Autodesk Inventor part; units mm, degrees
ref_plane "Work Plane1" through (-166.5525, 2.666, -98.7961) normal (0, 0, -1) x (-1, 0, 0)
ref_plane "Work Plane2" through (-38.4044, -9.834, -118.7961) normal (0, -1, 0) x (1, 0, 0)
ref_plane "Work Plane3" through (-25.7044, 2.666, -220.3961) normal (0, -1, 0) x (1, 0, 0)
ref_plane "Work Plane1" through (-166.5525, 2.666, -98.7961) normal (0, 0, -1) x (-1, 0, 0)
sketch "Sketch1" plane through (-166.5525, 2.666, -98.7961) normal (0, 0, -1) x (-1, 0, 0)
  line L0 (-233.1482, 205) -> (-133.1482, 205)
  line L1 (-133.1482, 205) -> (-133.1482, -25)
  line L2 (-133.1482, -25) -> (-233.1482, -25)
  line L3 (-233.1482, -25) -> (-233.1482, 205)
  circle A0 centre (0, 0) radius 140
  circle A1 centre (-210, 25) radius 2.4585
  circle A2 centre (-185, 25) radius 2.4585
  circle A3 centre (-160, 25) radius 2.4585
  circle A4 centre (-185, 0) radius 2.4585
  circle A5 centre (-210, 0) radius 2.4585
  circle A6 centre (-160, 0) radius 2.4585
  circle A7 centre (0.3518, 0) radius 128.5
  line L4 (-128.1482, 39.0483) -> (-128.1482, -22.9652) construction
  dimension "d10" = 5
  dimension "d56" = 230
  dimension "d57" = 100
  dimension "d63" = 25
extrude "Extrusion1" add sketch "Sketch1" along normal blind 10 contours L0 L1 A0 L2 L3 | L1 L2 A0 | A1 | A2 | A3 | A4 | A5 | A6 picked at (-134.3536, 16.0623)
hole "Hole1" at (43.4475, 27.666, -108.7961) at (18.4475, 27.666, -108.7961) at (-6.5525, 27.666, -108.7961) at (43.4475, 2.666, -108.7961) at (18.4475, 2.666, -108.7961) at (-6.5525, 2.666, -108.7961) direction (0, 0, 1) diameter 6.6 end through all counterbore diameter 11 counterbore depth 6.8
ref_plane "Work Plane2" through (-38.4044, -9.834, -118.7961) normal (0, -1, 0) x (1, 0, 0)
sketch "Sketch3" plane through (-38.4044, -9.834, -118.7961) normal (0, -1, 0) x (1, 0, 0)
  line L0 (5, 10) -> (55, 10)
  line L1 (55, 10) -> (55, -75)
  line L2 (50, -80) -> (32.7284, -80)
  line L3 (5, -35.6333) -> (5, 10)
  line L4 (105, 10) -> (5, 10)
  line L5 (5, 20) -> (5, 10)
  circle A0 centre (22.225, -22.225) radius 12.7
  circle A1 centre (22.225, -22.225) radius 10
  line L6 (5.6699, -38.1333) -> (28.3983, -77.5)
  line L7 (5, -36.973) -> (50.4568, -36.973) construction
  arc A2 (28.3983, -77.5) -> (32.7284, -80) centre (32.7284, -75) ccw
  arc A3 (50, -80) -> (55, -75) centre (50, -75) ccw
  arc A4 (5, -35.6333) -> (5.6699, -38.1333) centre (10, -35.6333) ccw
  point P0 (38.4044, 118.7961)
  dimension "d11" = 20
  dimension "d13" = 60
  dimension "d14" = 5
  dimension "d58" = 90
  dimension "d60" = 50
extrude "Extrusion2" add sketch "Sketch3" along normal mid plane 10 contours L0 L1 A3 L2 A2 L6 A4 L3 | A0
ref_plane "Work Plane3" through (-25.7044, 2.666, -220.3961) normal (0, -1, 0) x (1, 0, 0)
mirror "Mirror1" about plane through (-25.7044, 2.666, -220.3961) normal (0, -1, 0) of "Extrusion2"
sketch "Sketch4" plane through (-166.5525, 2.666, -108.7961) normal (0, 0, -1) x (-1, 0, 0)
  line L0 (-133.1482, 205) -> (-133.1482, -25)
  line L1 (-133.1482, 32.5) -> (-183.1482, 32.5)
  line L2 (-183.1482, 32.5) -> (-183.1482, 42.5)
  line L3 (-183.1482, 42.5) -> (-133.1482, 42.5)
  line L4 (-133.1482, 42.5) -> (-133.1482, 32.5)
  line L5 (-183.1482, 17.5) -> (-183.1482, 7.5)
  circle A0 centre (-185, 25) radius 3.3
  line L6 (-160.8766, 17.5) -> (-178.1482, 17.5)
  point P0 (-166.5525, -2.666)
  dimension "d17" = 4.2
  dimension "d18" = 4.2
  dimension "d19" = 10
extrude "Extrusion3" add sketch "Sketch4" along normal blind 50 contours L0 L1 L2 L3
fillet "Fillet1" radius 5 2 edges at (-33.4044, 40.166, -158.7961) (16.5956, 40.166, -158.7961)
sketch "Sketch5" plane through (-33.4044, 45.166, -108.7961) normal (0, 1, 0) x (1, 0, 0)
  circle A0 centre (17.225, 32.225) radius 10
  point P0 (33.4044, -108.7961)
extrude "Extrusion4" cut sketch "Sketch5" against normal blind 15.75
ref_plane "Work Plane6" through (-16.1794, 92.1501, -148.7711) normal (0, -1, 0) x (0, 0, 1)
sketch "Sketch7" plane through (-16.1794, 92.1501, -148.7711) normal (0, -1, 0) x (0, 0, 1)
  line L0 (39.975, 17.225) -> (39.975, -82.775)
  line L1 (39.975, 17.225) -> (-5.025, 17.225)
  line L2 (-10.025, 12.225) -> (-10.025, -12.775)
  line L3 (-5.025, -17.775) -> (39.975, -17.775)
  line L4 (39.975, -17.775) -> (39.975, 17.225)
  arc A0 (-5.025, 17.225) -> (-10.025, 12.225) centre (-5.025, 12.225) ccw
  arc A1 (-10.025, -12.775) -> (-5.025, -17.775) centre (-5.025, -12.775) ccw
  point P0 (148.7711, -16.1794)
  point P1 (-10.025, -17.775)
  point P2 (-10.025, 17.225)
  point P3 (7.75, 0)
  dimension "d25" = 50
  dimension "d26" = 35
  dimension "d27" = 5
extrude "Extrusion5" [suppressed]
sketch "Sketch8" plane through (-16.1794, 85.1501, -148.7711) normal (0, -1, 0) x (1, 0, 0)
  point P0 (16.1794, 148.7711)
  point P1 (0, 7.75)
hole "Hole2" [suppressed]
ref_plane "Work Plane8" through (-11.7294, 189.1501, -141.0211) normal (1, 0, 0) x (0, -1, 0)
sketch "Sketch12" plane through (-11.7294, 189.1501, -141.0211) normal (1, 0, 0) x (0, -1, 0)
  circle A0 centre (-2, 0) radius 2
  line L0 (0, 4.5164) -> (0, 7)
  line L1 (-9.233, 4.5164) -> (0, 4.5164)
  spline S0 degree 2 poles (-10, 3.4325) (-9.6688, 3.9374) (-9.233, 4.5164) knots 0 0 0 0.1328 0.1328 0.1328 weights 1 1.004688 1
  line L2 (-10, -3.4325) -> (-10, 3.4325)
  spline S1 degree 2 poles (-9.233, -4.5164) (-9.6688, -3.9374) (-10, -3.4325) knots 0 0 0 0.1328 0.1328 0.1328 weights 1 1.004688 1
  line L3 (0, -4.5164) -> (-9.233, -4.5164)
  line L4 (0, -7) -> (0, -4.5164)
  line L5 (0, -7) -> (4.2876, -7)
  spline S2 degree 2 poles (4, -6.6678) (4.1403, -6.8309) (4.2876, -7) knots 0 0 0 0.044596 0.044596 0.044596 weights 1 1.000378 1.000314
  line L6 (4, 6.6678) -> (4, -6.6678)
  spline S3 degree 2 poles (4.2876, 7) (4.1403, 6.8309) (4, 6.6678) knots 0.03161 0.03161 0.03161 0.076206 0.076206 0.076206 weights 1.000314 1.000378 1
  line L7 (-18.5159, -32.225) -> (211.4841, -32.225)
  line L8 (1.2341, 7.775) -> (-8.2659, 7.775)
  line L9 (-10.2659, 5.775) -> (-10.2659, -32.225)
  line L10 (-10.2659, -32.225) -> (3.2341, -32.225)
  line L11 (3.2341, -32.225) -> (3.2341, 5.775)
  arc A1 (-8.2659, 7.775) -> (-10.2659, 5.775) centre (-8.2659, 5.775) ccw
  arc A2 (3.2341, 5.775) -> (1.2341, 7.775) centre (1.2341, 5.775) ccw
  line L12 (-18.5159, -42.225) -> (-18.5159, -32.225)
  point P0 (189.1501, -141.0211)
  point P1 (3.2341, 7.775)
  point P2 (-3.5159, 7.775)
  dimension "d48" = 13.5
  dimension "d49" = 2
  dimension "d62" = 40
  dimension "d79" = 15
extrude "Extrusion7" add sketch "Sketch12" along normal blind 10
ref_plane "Work Plane10" through (-16.1794, 180.6501, -141.0211) normal (-1, 0, 0) x (0, 1, 0)
ref_plane "Work Plane9" through (-20.6294, 180.6501, -141.0211) normal (-1, 0, 0) x (0, 1, 0)
mirror "Mirror2" about plane through (-16.1794, 180.6501, -141.0211) normal (-1, 0, 0) of "Extrusion7"
sketch "Sketch13" plane through (-166.5525, 2.666, -108.7961) normal (0, 0, -1) x (-1, 0, 0)
  line L0 (-233.1482, 205) -> (-188.1482, 205)
  line L1 (-188.1482, 205) -> (-188.1482, 75)
  line L2 (-188.1482, 75) -> (-233.1482, 75)
  line L3 (-233.1482, 75) -> (-233.1482, 205)
  line L4 (-233.1482, -25) -> (-133.1482, -25)
  line L5 (-133.1482, 42.5) -> (-133.1482, 205)
  point P0 (-166.5525, -2.666)
  point P1 (-133.1482, 89.4841)
  dimension "d52" = 100
  dimension "d53" = 55
extrude "Extrusion8" [suppressed]
ref_plane "Work Plane11" through (-33.4044, 2.666, -108.7961) normal (0, -1, 0) x (1, 0, 0)
sketch "Sketch15" plane through (-166.5525, 2.666, -108.7961) normal (0, 0, -1) x (-1, 0, 0)
  line L0 (-133.1482, 205) -> (-133.1482, -25) construction
  line L1 (-133.1482, 95) -> (-183.1482, 95) construction
  line L2 (-133.1482, 95) -> (-83.1482, 95) construction
  line L3 (-133.1482, 205) -> (-233.1482, 205) construction
  line L4 (-183.1482, 91.5) -> (-133.1482, 91.5)
  line L5 (-133.1482, 91.5) -> (-133.1482, 98.5)
  line L6 (-133.1482, 98.5) -> (-183.1482, 98.5)
  line L7 (-183.1482, 98.5) -> (-183.1482, 91.5)
  line L8 (-183.1482, 91.5) -> (-133.1482, 98.5) construction
  line L9 (-133.1482, 91.5) -> (-183.1482, 98.5) construction
  point P0 (-166.5525, -2.666)
  point P1 (-158.1482, 95)
  dimension "d64" = 50
  dimension "d65" = 180
  dimension "d66" = 110
  dimension "d67" = 7
extrude "Extrusion9" add sketch "Sketch15" along normal blind 50
fillet "Fillet2" radius 5 2 edges at (-33.4044, 97.666, -158.7961) (16.5956, 97.666, -158.7961)
sketch "Sketch16" plane through (-33.4044, 101.166, -108.7961) normal (0, 1, 0) x (1, 0, 0)
  point P0 (33.4044, -108.7961)
  point P1 (17.225, 32.225)
hole "Hole3" at (-16.1794, 101.166, -141.0211) direction (0, -1, 0) diameter 12.2 depth 17.1 tip angle 118
equation "\"d18\" = d17"
properties part number "Verbinder_Tisch_Dewar"
Input: part model. Units: mm. Frame: model coordinates. A direction names the side the tool comes from. Coordinates: 2 decimals unless noted, no trailing zeros. Write each loop counter-clockwise with the first axis right and the second up, starting at its lowest first coordinate (ties: lowest second). Pieces come first, ordered by that corner, then holes. Notation, with made-up numbers: (44, 68) - (95, 68) arc R20 cw to (95, 101) - close; hole circle Ø2 at (-39, 88). An arc over 180 degrees is marked (long way). Put each result on its own line as item: value. Start each with the question number.
1) Mould query, pull axis Y, two halves, no side actions, for faces 6 (the face through (-3, -14.834, -153)), 7 (the face through (-8, 45.166, -133)), 8 (the face through (16.22, 0.23, -100.37)), 9 (the face through (-18.35, 40.24, -131.26)). Classes: pulls with the +Y half, pulls with the -Y half, needs draft (parallel to the pull), parting line crosses it, or undercut.
2) Cut plane C-C (x = 28). Return the cut outline in (y, z), plus the area to 3 significant figures.
3) Ray query, L1, parallel to Y at x = 5.5, z = -131; L2, parallel to Y at x = -7.5, z = -192; L3, parallel to X at y = 192, z = -147. Return the intervals inside material, ascending.
4) Contact query for flat-ended pins moving along their axis: pin 1 (10 mm diameter, centred on x = 50.5, y = 42, fed in from -Z); pin 2 (4 mm diameter, centred on y = 194, z = -120.5, fed in from -X); pin 3 (25 mm diameter, centred on x = -15.5, z = -123, fed in from +Y). Output: stop coordinate, or through.
5) Cut plane A-A (z = -125.5). Return the cut outline in (x, y), plus the area to 3 significant figures.
6) Reachability of faces 1 (the face through (-30.629, 193, -129)), 2 (the face through (46.79, -1.7, -105.35)), 3 (the face through (-18.35, 15.24, -131.26)), 4 (the face through (15.09, 97.62, -157.37)), 5 (the face through (-20.629, 193, -129)) from +Z, -Z, +X, -X, +Y, -Y: full face, straight path, thin tool, end or side. Return the list, or none.
7) Cut plane B-B (z = -189). Return the cut outline in (x, y), plus the area to 3 significant figures.
8) Cut plane D-D (z = -169). Return the cut outline in (x, y), plus the area to 3 significant figures.
Resolved:
1. face 6: pulls with the -Y half
1. face 7: undercut
1. face 8: undercut
1. face 9: needs draft
2. outline: (-22.33, -108.8) - (207.67, -108.8) - (207.67, -98.8) - (-22.33, -98.8) - close
2. area: 2,300 mm2
3. L1: y = -14.83 to -4.83, 10.17 to 20.17, 35.17 to 45.17, 94.17 to 101.17
3. L2: y = -14.83 to -4.83, 10.17 to 20.17
3. L3: x = -30.63 to -20.63, -11.73 to -1.73
4. pin 1: stops at z = -108.8
4. pin 2: stops at x = -30.63
4. pin 3: stops at y = 199.42
5. outline: (-33.4, -14.83) - (16.6, -14.83) - (16.6, -4.83) - (-33.4, -4.83) - close; (-33.4, 10.17) - (16.6, 10.17) - (16.6, 20.17) - (-33.4, 20.17) - close; (-33.4, 35.17) - (16.6, 35.17) - (16.6, 45.17) - (-33.4, 45.17) - close; (-33.4, 94.17) - (16.6, 94.17) - (16.6, 101.17) - (-33.4, 101.17) - close; (-30.63, 185.92) - (-20.63, 185.92) - (-20.63, 199.42) - (-30.63, 199.42) - close; (-11.73, 185.92) - (-1.73, 185.92) - (-1.73, 199.42) - (-11.73, 199.42) - close
5. area: 2,120 mm2
6. face 1: -Z, -X, +Y
6. face 2: -Z
6. face 3: -Y
6. face 4: -Z, +X, +Y
6. face 5: -Z, +Y
7. outline: (-14.22, -14.83) - (16.6, -14.83) - (16.6, -4.83) - (-14.22, -4.83) - close; (-14.22, 10.17) - (16.6, 10.17) - (16.6, 20.17) - (-14.22, 20.17) - close
7. area: 616 mm2
8. outline: (-25.77, -14.83) - (16.6, -14.83) - (16.6, -4.83) - (-25.77, -4.83) - close; (-25.77, 10.17) - (16.6, 10.17) - (16.6, 20.17) - (-25.77, 20.17) - close
8. area: 847 mm2
